Can you work these out from the model? Positions are in its coordinate system, mm. A direction names the side the tool comes from. Give positions to 0.01 mm unless a question says otherwise; leave off trailing zeros. Loops run counter-clockwise (first coordinate to the right, second up) from the corner with the lowest first, then second, coordinate; pieces in that order, holes last. Notation, with made-up numbers: (28, -17) -> (87, -17) arc R22 ccw to (87, -11) -> close; hole circle Ø1 at (9, 6). An arc over 180 degrees is marked (long way). One line per question, with ' | ' between items.
from build123d import *

# Parameters (mm, degrees)
EXTRUDE_1_DEPTH              = 212
SKETCH_2_W                   = 38.1
SKETCH_2_H                   = 16
CUT_EXTRUDE_1_DEPTH          = 23
HOLE_WIZARD_M31_AT_2_COUNT   = 2
HOLE_WIZARD_M31_AT_2_PITCH   = 48
HOLE_WIZARD_M31_AT_3_COUNT   = 2
HOLE_WIZARD_M31_AT_3_PITCH   = 66.753277073
HOLE_WIZARD_M31_AT_4_COUNT   = 2
HOLE_WIZARD_M31_AT_4_PITCH   = 42
HOLE_WIZARD_M31_AT_5_COUNT   = 2
HOLE_WIZARD_M31_AT_5_PITCH   = 43.17406629
HOLE_WIZARD_M31_AT_6_COUNT   = 2
HOLE_WIZARD_M31_AT_6_PITCH   = 96.519428096
HOLE_WIZARD_M31_AT_7_COUNT   = 2
HOLE_WIZARD_M31_AT_7_PITCH   = 96
HOLE_WIZARD_M31_AT_8_COUNT   = 2
HOLE_WIZARD_M31_AT_8_PITCH   = 10
HOLE_WIZARD_M31_AT_9_COUNT   = 2
HOLE_WIZARD_M31_AT_9_PITCH   = 49.030602689
HOLE_WIZARD_M31_2_AT_2_COUNT = 2
HOLE_WIZARD_M31_2_AT_2_PITCH = 13
HOLE_WIZARD_M31_2_AT_3_COUNT = 2
HOLE_WIZARD_M31_2_AT_3_PITCH = 190.510498398
HOLE_WIZARD_M32_AT_2_COUNT   = 2
HOLE_WIZARD_M32_AT_2_PITCH   = 50
HOLE_WIZARD_M32_AT_3_COUNT   = 2
HOLE_WIZARD_M32_AT_3_PITCH   = 110
HOLE_WIZARD_M32_AT_4_COUNT   = 2
HOLE_WIZARD_M32_AT_4_PITCH   = 160


with BuildPart() as part:
    # Эскиз1 → Бобышка-Вытянуть1 (new body)
    with BuildSketch(Plane.XY):
        Polygon((-20, 20), (-20, 0), (20, 0), (20, 22), (18.1, 22), (18.1, 1.9), (-18.1, 1.9), (-18.1, 20), align=None)
    extrude(amount=EXTRUDE_1_DEPTH)

    # Эскиз2 → Вырез-Вытянуть1 (cut, through all)
    with BuildSketch(Plane(origin=(0, 0, 0), x_dir=(1, 0, 0), z_dir=(0, 1, 0))):
        with Locations((-0.95, -204)):
            Rectangle(SKETCH_2_W, SKETCH_2_H)
        with Locations((-0.95, -8)):
            Rectangle(SKETCH_2_W, SKETCH_2_H)
    extrude(amount=CUT_EXTRUDE_1_DEPTH, mode=Mode.SUBTRACT)

    # Эскиз4 → Hole Wizard M31 (revolve, cut)
    with BuildSketch(Plane(origin=(-18.1, 6, 91), x_dir=(0, 0, -1), z_dir=(0, 1, 0))):
        Polygon((0, 0), (0, 1.9), (1.9, 1.9), (1.8, 1.8), (1.8, 1.2), (3, 0), align=None)
    hole_wizard_m31 = revolve(axis=Axis((-11.75, 6, 91), (-1, 0, 0)), mode=Mode.SUBTRACT)

    # Hole Wizard M31 at 2: Hole Wizard M31 ×2
    with Locations(*[(0, 0, -i * HOLE_WIZARD_M31_AT_2_PITCH) for i in range(1, HOLE_WIZARD_M31_AT_2_COUNT)]):
        add(hole_wizard_m31, mode=Mode.SUBTRACT)

    # Hole Wizard M31 at 3: Hole Wizard M31 ×2
    with Locations(*[Vector(0, 0.149805379, -0.988715504) * (i * HOLE_WIZARD_M31_AT_3_PITCH) for i in range(1, HOLE_WIZARD_M31_AT_3_COUNT)]):
        add(hole_wizard_m31, mode=Mode.SUBTRACT)

    # Hole Wizard M31 at 4: Hole Wizard M31 ×2
    with Locations(*[(0, 0, i * HOLE_WIZARD_M31_AT_4_PITCH) for i in range(1, HOLE_WIZARD_M31_AT_4_COUNT)]):
        add(hole_wizard_m31, mode=Mode.SUBTRACT)

    # Hole Wizard M31 at 5: Hole Wizard M31 ×2
    with Locations(*[Vector(0, 0.231620527, 0.972806215) * (i * HOLE_WIZARD_M31_AT_5_PITCH) for i in range(1, HOLE_WIZARD_M31_AT_5_COUNT)]):
        add(hole_wizard_m31, mode=Mode.SUBTRACT)

    # Hole Wizard M31 at 6: Hole Wizard M31 ×2
    with Locations(*[Vector(0, 0.103606084, 0.994618409) * (i * HOLE_WIZARD_M31_AT_6_PITCH) for i in range(1, HOLE_WIZARD_M31_AT_6_COUNT)]):
        add(hole_wizard_m31, mode=Mode.SUBTRACT)

    # Hole Wizard M31 at 7: Hole Wizard M31 ×2
    with Locations(*[(0, 0, i * HOLE_WIZARD_M31_AT_7_PITCH) for i in range(1, HOLE_WIZARD_M31_AT_7_COUNT)]):
        add(hole_wizard_m31, mode=Mode.SUBTRACT)

    # Hole Wizard M31 at 8: Hole Wizard M31 ×2
    with Locations(*[(0, i * HOLE_WIZARD_M31_AT_8_PITCH, 0) for i in range(1, HOLE_WIZARD_M31_AT_8_COUNT)]):
        add(hole_wizard_m31, mode=Mode.SUBTRACT)

    # Hole Wizard M31 at 9: Hole Wizard M31 ×2
    with Locations(*[Vector(0, 0.203954254, -0.97898042) * (i * HOLE_WIZARD_M31_AT_9_PITCH) for i in range(1, HOLE_WIZARD_M31_AT_9_COUNT)]):
        add(hole_wizard_m31, mode=Mode.SUBTRACT)

    # Эскиз7 → Hole Wizard M31 2 (revolve, cut)
    with BuildSketch(Plane(origin=(20, 2, 202.5), x_dir=(0, 0, -1), z_dir=(0, 1, 0))):
        Polygon((0, 0), (0, 1.9), (1.7, 1.9), (1.6, 1.8), (1.6, 0.1), (1.7, 0), align=None)
    hole_wizard_m31_2 = revolve(axis=Axis((26.35, 2, 202.5), (-1, 0, 0)), mode=Mode.SUBTRACT)

    # Hole Wizard M31 2 at 2: Hole Wizard M31 2 ×2
    with Locations(*[(0, i * HOLE_WIZARD_M31_2_AT_2_PITCH, 0) for i in range(1, HOLE_WIZARD_M31_2_AT_2_COUNT)]):
        add(hole_wizard_m31_2, mode=Mode.SUBTRACT)

    # Hole Wizard M31 2 at 3: Hole Wizard M31 2 ×2
    with Locations(*[Vector(0, 0.010498109, -0.999944893) * (i * HOLE_WIZARD_M31_2_AT_3_PITCH) for i in range(1, HOLE_WIZARD_M31_2_AT_3_COUNT)]):
        add(hole_wizard_m31_2, mode=Mode.SUBTRACT)

    # Эскиз9 → Зенковка для винта с потайной головкой M32 (revolve, cut)
    with BuildSketch(Plane(origin=(12.2, 1.9, 186), x_dir=(0, 0, 1), z_dir=(1, 0, 0))):
        Polygon((0, 0), (0, 1.9), (1.9, 1.9), (1.8, 1.8), (1.8, 1.2), (3, 0), align=None)
    hole_wizard_m32 = revolve(axis=Axis((12.2, 8.25, 186), (0, -1, 0)), mode=Mode.SUBTRACT)

    # Зенковка для винта с потайной головкой M32 at 2: Зенковка для винта с потайной головкой M32 ×2
    with Locations(*[(0, 0, -i * HOLE_WIZARD_M32_AT_2_PITCH) for i in range(1, HOLE_WIZARD_M32_AT_2_COUNT)]):
        add(hole_wizard_m32, mode=Mode.SUBTRACT)

    # Зенковка для винта с потайной головкой M32 at 3: Зенковка для винта с потайной головкой M32 ×2
    with Locations(*[(0, 0, -i * HOLE_WIZARD_M32_AT_3_PITCH) for i in range(1, HOLE_WIZARD_M32_AT_3_COUNT)]):
        add(hole_wizard_m32, mode=Mode.SUBTRACT)

    # Зенковка для винта с потайной головкой M32 at 4: Зенковка для винта с потайной головкой M32 ×2
    with Locations(*[(0, 0, -i * HOLE_WIZARD_M32_AT_4_PITCH) for i in range(1, HOLE_WIZARD_M32_AT_4_COUNT)]):
        add(hole_wizard_m32, mode=Mode.SUBTRACT)


solid = part.part
Q1. If we section it at C-C (x = -9): Write out the boundary of the cut face in (y, z), plus the area to 3 significant figures.
Entries:
outline: (0, 16) -> (1.9, 16) -> (1.9, 196) -> (0, 196) -> close | area: 342 mm²
Q2. If we section it at B-B (z = 120.5): Write out the boundary of the cut face in (x, y), plus the area to 3 significant figures.
Entries:
outline: (-20, 0) -> (20, 0) -> (20, 22) -> (18.1, 22) -> (18.1, 1.9) -> (-18.1, 1.9) -> (-18.1, 20) -> (-20, 20) -> close | area: 149 mm²
Q3. On a 3-axis mill with a long thin cutter (end or side, diameter ignored), from which of +Z, -Z, +X, -X, +Y, -Y can I reach the whole of each face in a straight line? I mean faces 4 (the face through (-19.6, 15.92, 92.8)), 5 (the face through (10.983, 0.404, 134.673)). Say none if no direction works.
Entries:
face 4: -X | face 5: +Y, -Y
Q4. For pin 1 Ø1.5 at (x, z) = (15, 73) entering from +Y; pin 2 Ø2 at (y, z) = (6, 133) entering from -X; pin 3 Ø4 at (x, z) = (9.5, 92.5) entering from -Y; pin 4 Ø0.9 at (x, z) = (-19, 120.5) entering from +Y, each with a flat end and sliding along its axis, tell me the tip position at first contact or that it passes through.
Entries:
pin 1: y = 1.9 | pin 2: x = 18.1 | pin 3: y = 0 | pin 4: y = 20
Q5. If I drill on probe 1 along Y at (x, z) = (-19.7, 187); probe 2 along Z at (x, y) = (-19.4, 6); probe 3 along Z at (x, y) = (-19.4, 16), over which ranges is the centre line in solid material (lowest first)? Write a range as from..to.
Entries:
probe 1: 0..4.2, 7.8..14.2, 17.8..20 | probe 2: 16..41.2, 44.8..89.2, 92.8..131.2, 134.8..185.2, 188.8..196 | probe 3: 16..23.2, 26.8..41.2, 44.8..89.2, 92.8..131.2, 134.8..185.2, 188.8..196
Q6. If we section it at A-A (z = 76): Write out the boundary of the cut face in (x, y).
Entries:
outline: (-20, 0) -> (10.3, 0) -> (10.4, 0.1) -> (10.4, 0.7) -> (9.2, 1.9) -> (-18.1, 1.9) -> (-18.1, 20) -> (-20, 20) -> close; (14, 0.1) -> (14.1, 0) -> (20, 0) -> (20, 22) -> (18.1, 22) -> (18.1, 1.9) -> (15.2, 1.9) -> (14, 0.7) -> close
Q7. If we mould it in two halves opening along Z, with no side actions, what happens to faces 1 (the face through (0, 0, 105)), 2 (the face through (-7, 1, 16)), 3 (the face through (11.659, 0.404, 27.717))? For each: pulls with the +Z half, pulls with the -Z half, needs draft (parallel to the pull), parting line crosses it, or undercut.
Entries:
face 1: needs draft | face 2: pulls with the -Z half | face 3: undercut
